Read the model definition and answer for the solid it produces. Units are mm, in the model's axes. A direction names the side the tool comes from. Round coordinates to 2 decimals unless told otherwise and drop trailing zeros. Order: outer loops, then holes, each group sorted by start corner. A loop starts at its lowest first (then second) coordinate and runs counter-clockwise, first axis right, second up. Notation, with made-up numbers: (7, 52) -> (21, 52) arc R22 cw to (21, 73) -> close; hole circle Ø4 at (70, -0.5). An arc over 180 degrees is marked (long way). One line per item, written item: value. Start each with the question number.
1. Flat-ended cylindrical pins translate along their axes: pin 1 Ø8 at (x, z) = (-2, -9.5) entering from +Y; pin 2 Ø4 at (x, y) = (-1, 8) entering from +Z; pin 3 Ø2 at (x, y) = (2, 6.5) entering from -Z. Find the tip coordinate at first contact, or state that the pin passes through.
2. For faces 1 (the face through (-3.4, 6.5, -1.4)), 2 (the face through (4.25, 5, 2)), 3 (the face through (0, 5, 6.1)), determine the directions among +Z, -Z, +X, -X, +Y, -Y from which every point of the face is accessible in a straight line to the end or side of a thin tool.
3. Section C-C (y = 7) is taken. Give the vertices of the cut face in (x, z), then the cut area to 3 significant figures.
4. Section D-D (z = -7.75) is taken. Give the vertices of the cut face in (x, y), then the cut area to 3 significant figures.
5. Consider line 1 (X direction, y = 4, z = -0.5); line 2 (Y direction, x = 4, z = -5); line 3 (Z direction, x = -2.75, y = 6). Determine where each line is inside the solid, lowest interval first.
6. Section B-B (x = 2) is taken. Give the vertices of the cut face in (y, z), then the cut area to 3 significant figures.
7. Section A-A (z = 5.25) is taken. Give the vertices of the cut face in (x, y).
from build123d import *

# Parameters (mm, degrees)
SKETCH1_W           = 25
SKETCH1_H           = 23.8
BOSS_EXTRUDE1_DEPTH = 3.5
BOSS_EXTRUDE2_START = -3.5
SKETCH2_W           = 8.5
SKETCH2_H           = 8.5
BOSS_EXTRUDE2_DEPTH = 6.5
BOSS_EXTRUDE3_START = -6.5
SKETCH3_R           = 4.25
BOSS_EXTRUDE3_DEPTH = 9


with BuildPart() as part:
    # Sketch1 → Boss-Extrude1 (new body)
    with BuildSketch(Plane(origin=(0, 0, 0), x_dir=(1, 0, 0), z_dir=(0, 1, 0))):
        Rectangle(SKETCH1_W, SKETCH1_H)
    extrude(amount=BOSS_EXTRUDE1_DEPTH)

    # Sketch2 → Boss-Extrude2 (add)
    with BuildSketch(Plane(origin=(0, 3.5, 0), x_dir=(1, 0, 0), z_dir=(0, 1, 0)).offset(BOSS_EXTRUDE2_START)):
        with Locations((0, -1.85)):
            Rectangle(SKETCH2_W, SKETCH2_H)
    extrude(amount=BOSS_EXTRUDE2_DEPTH)

    # Sketch3 → Boss-Extrude3 (add)
    with BuildSketch(Plane(origin=(0, 6.5, 0), x_dir=(1, 0, 0), z_dir=(0, 1, 0)).offset(BOSS_EXTRUDE3_START)):
        with Locations((0, -1.85)):
            Circle(SKETCH3_R)
    extrude(amount=BOSS_EXTRUDE3_DEPTH)


solid = part.part
Answer:
1. pin 1: y = 3.5
1. pin 2: z = 6.1
1. pin 3: z = -2.4
2. face 1: -Z, -X, +Y
2. face 2: +Z, -Z, +X, +Y
2. face 3: +Z, +X, -X, +Y
3. outline: circle Ø8.5 at (0, 1.85)
3. area: 56.7 mm^2
4. outline: (-12.5, 0) -> (12.5, 0) -> (12.5, 3.5) -> (-12.5, 3.5) -> close
4. area: 87.5 mm^2
5. line 1: -4.25 to 4.25
5. line 2: 0 to 3.5
5. line 3: -2.4 to 6.1
6. outline: (0, -11.9) -> (3.5, -11.9) -> (3.5, -2.4) -> (6.5, -2.4) -> (6.5, -1.9) -> (9, -1.9) -> (9, 5.6) -> (6.5, 5.6) -> (6.5, 6.1) -> (3.5, 6.1) -> (3.5, 11.9) -> (0, 11.9) -> close
6. area: 128 mm^2
7. outline: (-12.5, 0) -> (12.5, 0) -> (12.5, 3.5) -> (4.25, 3.5) -> (4.25, 6.5) -> (2.55, 6.5) -> (2.55, 9) -> (-2.55, 9) -> (-2.55, 6.5) -> (-4.25, 6.5) -> (-4.25, 3.5) -> (-12.5, 3.5) -> close
